from build123d import *

# Parameters (mm, degrees)
F1_DEPTH = 5.08
F2_R     = 0.508
F3_R     = 0.508
F5_DEPTH = 2.54


with BuildPart() as f1:
    # F0 (on Top) → F1 (new body)
    with BuildSketch(Plane.XY):
        with BuildLine():
            ThreePointArc((-29.131383, -4.682618), (-16.468234, -4.474505), (-4.436489, -8.428712))
            ThreePointArc((-4.436489, -8.428712), (-2.284966, -9.246867), (0, -9.525))
            ThreePointArc((0, -9.525), (2.284966, -9.246867), (4.436489, -8.428712))
            ThreePointArc((4.436489, -8.428712), (16.468234, -4.474505), (29.131383, -4.682618))
            ThreePointArc((29.131383, -4.682618), (34.7625, 0), (29.131383, 4.682618))
            ThreePointArc((29.131383, 4.682618), (16.468234, 4.474505), (4.436489, 8.428712))
            ThreePointArc((4.436489, 8.428712), (2.284966, 9.246867), (0, 9.525))
            ThreePointArc((0, 9.525), (-2.284966, 9.246867), (-4.436489, 8.428712))
            ThreePointArc((-4.436489, 8.428712), (-16.468234, 4.474505), (-29.131383, 4.682618))
            ThreePointArc((-29.131383, 4.682618), (-34.7625, 0), (-29.131383, -4.682618))
        make_face()
        Polygon((-4.05, 2.338269), (0, 4.676537), (4.05, 2.338269), (4.05, -2.338269), (0, -4.676537), (-4.05, -2.338269), align=None, mode=Mode.SUBTRACT)
    extrude(amount=F1_DEPTH)

    # F2
    f2_edges = [f1.edges().sort_by_distance(p)[0] for p in [
        (-34.7625, 0, 5.08),
        (-16.468234, -4.474505, 5.08),
        (0, -9.525, 5.08),
        (16.468234, -4.474505, 5.08),
        (34.7625, 0, 5.08),
        (16.468234, 4.474505, 5.08),
        (0, 9.525, 5.08),
        (-16.468234, 4.474505, 5.08),
        (-2.025, 3.507403, 5.08),
        (2.025, 3.507403, 5.08),
        (4.05, 0, 5.08),
        (2.025, -3.507403, 5.08),
        (-2.025, -3.507403, 5.08),
        (-4.05, 0, 5.08),
    ]]
    fillet(f2_edges, radius=F2_R)

    # F3
    f3_edges = [f1.edges().sort_by_distance(p)[0] for p in [
        (-34.7625, 0, 0),
        (-16.468234, -4.474505, 0),
        (0, -9.525, 0),
        (16.468234, -4.474505, 0),
        (34.7625, 0, 0),
        (16.468234, 4.474505, 0),
        (0, 9.525, 0),
        (-16.468234, 4.474505, 0),
        (-2.025, 3.507403, 0),
        (2.025, 3.507403, 0),
        (4.05, 0, 0),
        (2.025, -3.507403, 0),
        (-2.025, -3.507403, 0),
        (-4.05, 0, 0),
    ]]
    fillet(f3_edges, radius=F3_R)

    # F4 (on face) → F5 (cut)
    with BuildSketch(Plane.XY.offset(5.08)):
        with BuildLine():
            ThreePointArc((29.687298, -1.685742), (31.7145, 0), (29.687298, 1.685742))
            ThreePointArc((29.687298, 1.685742), (18.897854, 1.126865), (8.334847, 3.395633))
            ThreePointArc((8.334847, 3.395633), (9, 0), (8.334847, -3.395633))
            ThreePointArc((8.334847, -3.395633), (18.897854, -1.126865), (29.687298, -1.685742))
        make_face()
        with BuildLine():
            ThreePointArc((-8.334847, -3.395633), (-9, 0), (-8.334847, 3.395633))
            ThreePointArc((-8.334847, 3.395633), (-18.897854, 1.126865), (-29.687298, 1.685742))
            ThreePointArc((-29.687298, 1.685742), (-31.7145, 0), (-29.687298, -1.685742))
            ThreePointArc((-29.687298, -1.685742), (-18.897854, -1.126865), (-8.334847, -3.395633))
        make_face()
    extrude(amount=-F5_DEPTH, mode=Mode.SUBTRACT)


solid = f1.part
The model under review builds one solid part; all positions refer to its coordinate system, in mm. A direction names the side the tool comes from. Coordinates: 2 decimals unless noted, no trailing zeros. Loops run counter-clockwise (first coordinate to the right, second up) from the corner with the lowest first, then second, coordinate; pieces in that order, holes last. Notation, with made-up numbers: (67, 53.5) -> (83, 53.5) arc R7 cw to (83, 59.5) -> close; hole circle Ø2 at (-4.75, 44). An arc over 180 degrees is marked (long way). Use a Markdown table: item, result. Add a question column.
1. Clearance check with flat-ended pins moving along their axes: pin 1 Ø1.5 at (x, y) = (-12.5, 7) entering from -Z; pin 2 Ø1.2 at (y, z) = (1, 2) entering from +X; pin 3 Ø3 at (x, y) = (30, 0) entering from +Z; pin 4 Ø5 at (x, y) = (9.5, -1.5) entering from -Z. State where each tip first meets the part, or that it passes through.
2. Add section A-A on y = 0. Write out the cut boundary in (x, z).
3. To check wall thickness, follow line 1 (X direction, y = 0, z = 3.3); line 2 (Y direction, x = 30, z = 3.15); line 3 (X direction, y = 3.75, z = 2). State the ranges of each line that lie inside material, in increasing order.
4. Machinability: for faces 1 (the face through (2.1, -3.7, 0.1)), 2 (the face through (2.053, -3.491, 2.512)), 3 (the face through (-31.714, 0.042, 3.828)), 4 (the face through (-16.3, 4.5, 2.5)), 5 (the face through (-16.64, -4.45, 2.51)), which of the approach directions +Z, -Z, +X, -X, +Y, -Y give a long, thin tool a straight path to every point of the face, cutting with its end or side? Answer none if there is none.
Returned:
| question | item | result |
|---|---|---|
| 1 | pin 1 | passes through |
| 1 | pin 2 | stops at x = 34.75 |
| 1 | pin 3 | stops at z = 2.54 |
| 1 | pin 4 | stops at z = 0 |
| 2 | outline | (-34.76, 0.51) arc R0.51 ccw to (-34.25, 0) -> (-4.56, 0) arc R0.51 ccw to (-4.05, 0.51) -> (-4.05, 4.57) arc R0.51 ccw to (-4.56, 5.08) -> (-9, 5.08) -> (-9, 2.54) -> (-31.71, 2.54) -> (-31.71, 5.08) -> (-34.25, 5.08) arc R0.51 ccw to (-34.76, 4.57) -> close; (4.05, 0.51) arc R0.51 ccw to (4.56, 0) -> (34.25, 0) arc R0.51 ccw to (34.76, 0.51) -> (34.76, 4.57) arc R0.51 ccw to (34.25, 5.08) -> (31.71, 5.08) -> (31.71, 2.54) -> (9, 2.54) -> (9, 5.08) -> (4.56, 5.08) arc R0.51 ccw to (4.05, 4.57) -> close |
| 3 | line 1 | x = -34.76 to -31.71, -9 to -4.05, 4.05 to 9, 31.71 to 34.76 |
| 3 | line 2 | y = -4.76 to -1.71, 1.71 to 4.76 |
| 3 | line 3 | x = -32.94 to -1.6, 1.6 to 32.94 |
| 4 | face 1 | -Z |
| 4 | face 2 | +Z, -Z |
| 4 | face 3 | +Z |
| 4 | face 4 | +Z, -Z, +Y |
| 4 | face 5 | +Z, -Z, -Y |
